Geometry: see drawing. Coordinates: mm, zero at the bounding-box minimum. A direction names the side the tool comes from. Coordinates: 2 decimals unless noted, no trailing zeros. Order: outer loops, then holes, each group sorted by start corner. A loop starts at its lowest first (then second) coordinate and runs counter-clockwise, first axis right, second up.
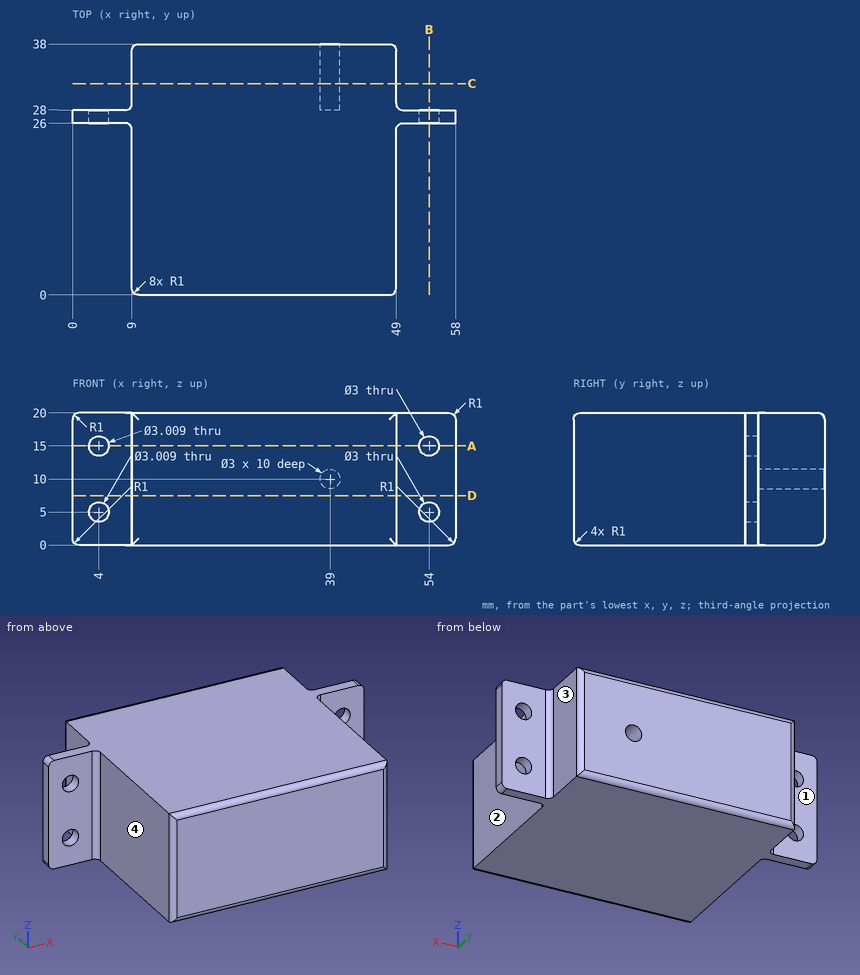
Q1. Pin query (flat end, axial travel): P1, Ø8, axis at y = 11.5, z = 3.5, coming from the -X side; P2, Ø5, axis at x = 4, z = 15, coming from the -Y side; P3, Ø2.5, axis at x = 54, z = 5, coming from the -Y side; P4, Ø10, axis at y = 17, z = 14.5, coming from the +X side. Return the tip coordinate at first contact, or that it passes through.
Solutions:
P1: stops at x = 9
P2: stops at y = 26
P3: passes through
P4: stops at x = 49
Q2. Material intervals for line 1 along X through (y, z) = (26.6, 15) (1 decimal); line 2 along Z through (x, y) = (3.5, 26.5); line 3 along X through (y, z) = (27.5, 14) (1 decimal), sorted ascending.
Solutions:
line 1: x = 0 to 2.5, 5.5 to 52.5, 55.5 to 58
line 2: z = 0 to 3.58, 6.42 to 13.58, 16.42 to 20
line 3: x = 0 to 2.9, 5.1 to 52.9, 55.1 to 58
Q3. Section query C-C on y = 32. Output: boundary loops of the cut face in (x, z), plus the area to 3 significant figures.
Solutions:
outline: (9, 0) - (49, 0) - (49, 20) - (9, 20) - close; hole circle Ø3 at (39, 10)
area: 793 mm2
Q4. Set-up query: the marked faces 1, 2, 3 and 4. Return all of +Z, -Z, +X, -X, +Y, -Y with unobstructed straight access to the full face (end or side cutting, diameter ignored); none if empty.
Solutions:
face 1: +Z, -Z, -X, +Y
face 2: +Z, -Z, +X, -Y
face 3: +Z, -Z, +X, +Y
face 4: +Z, -Z, -X, -Y
Q5. Section query D-D on z = 7.5. Output: boundary loops of the cut face in (x, y).
Solutions:
outline: (0, 26) - (8, 26) arc R1 cw to (9, 25) - (9, 1) arc R1 ccw to (10, 0) - (48, 0) arc R1 ccw to (49, 1) - (49, 25) arc R1 cw to (50, 26) - (58, 26) - (58, 28) - (50, 28) arc R1 cw to (49, 29) - (49, 37) arc R1 ccw to (48, 38) - (10, 38) arc R1 ccw to (9, 37) - (9, 29) arc R1 cw to (8, 28) - (0, 28) - close
Q6. Section query A-A on z = 15. Output: boundary loops of the cut face in (x, y) (1 decimal).
Solutions:
outline: (0, 26) - (2.5, 26) - (2.5, 28) - (0, 28) - close; (5.5, 26) - (8, 26) arc R1 cw to (9, 25) - (9, 1) arc R1 ccw to (10, 0) - (48, 0) arc R1 ccw to (49, 1) - (49, 25) arc R1 cw to (50, 26) - (52.5, 26) - (52.5, 28) - (50, 28) arc R1 cw to (49, 29) - (49, 37) arc R1 ccw to (48, 38) - (10, 38) arc R1 ccw to (9, 37) - (9, 29) arc R1 cw to (8, 28) - (5.5, 28) - close; (55.5, 26) - (58, 26) - (58, 28) - (55.5, 28) - close
Q7. Section query B-B on x = 54. Output: boundary loops of the cut face in (y, z), plus the area to 3 significant figures.
Solutions:
outline: (26, 0) - (28, 0) - (28, 3.5) - (26, 3.5) - close; (26, 6.5) - (28, 6.5) - (28, 13.5) - (26, 13.5) - close; (26, 16.5) - (28, 16.5) - (28, 20) - (26, 20) - close
area: 28.0 mm2
